Source: three-view drawing plus pictorial views. Frame: mm from the lowest corner of the part. A direction names the side the tool comes from. Coordinates: 2 decimals unless noted, no trailing zeros. Order: outer loops, then holes, each group sorted by start corner. A loop starts at its lowest first (then second) coordinate and runs counter-clockwise, first axis right, second up. Notation, with made-up numbers: (22.5, 21) - (44.5, 21) arc R21 cw to (44.5, 48) - close; hole circle Ø3 at (14, 87). An arc over 180 degrees is marked (long way). One line per question, with ' | ' between items.
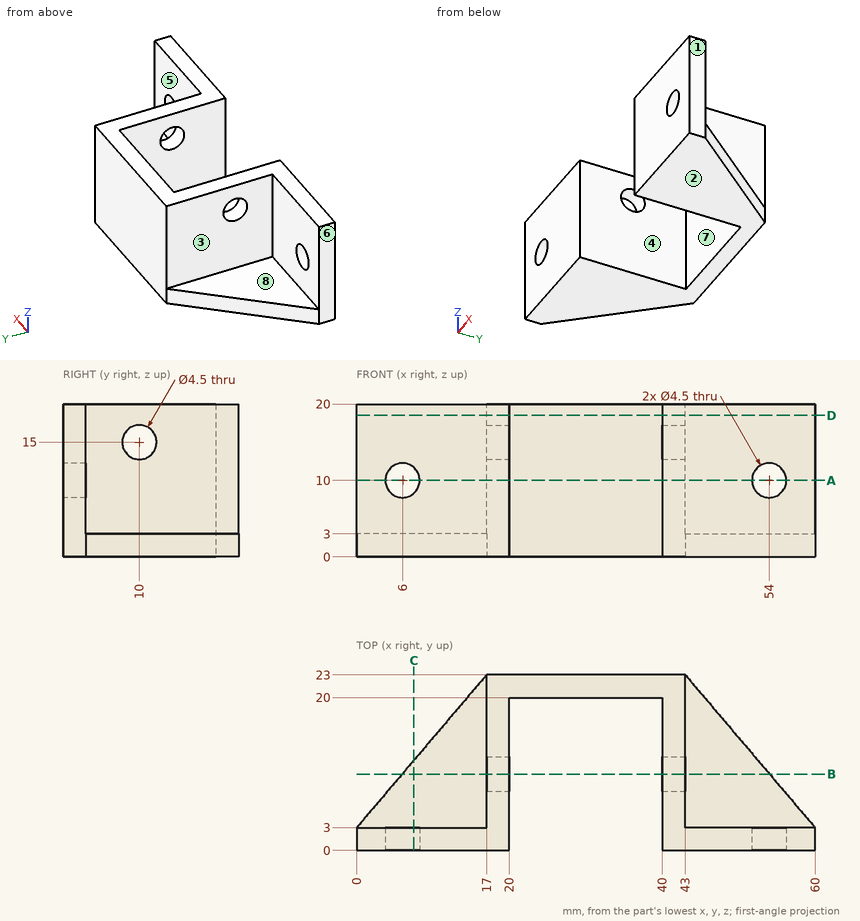
Item 1: Ray query, line 1 (X direction, y = 0.9, z = 10); line 2 (X direction, y = 8.75, z = 11.5); line 3 (Y direction, x = 40.75, z = 15). Return the intervals inside material, ascending.
Data:
line 1: 0 to 3.75, 8.25 to 20, 40 to 51.75, 56.25 to 60 | line 2: 17 to 20, 40 to 43 | line 3: 0 to 7.75, 12.25 to 23
Item 2: Access query for the marked faces 5, 6, 7 and 8. Directions: +Z, -Z, +X, -X, +Y, -Y. A direction counts if a zero-diameter tool reaches every point of the face in a straight line with its end or side. Return the directions, or none.
Data:
face 5: +Z, +X, +Y | face 6: +Z, -Z, -X, +Y, -Y | face 7: +Z, -Z, -Y | face 8: +Z, -X, +Y
Item 3: Section A-A on z = 10. Return the cut outline in (x, y).
Data:
outline: (0, 0) - (3.75, 0) - (3.75, 3) - (0, 3) - close; (8.25, 0) - (20, 0) - (20, 20) - (40, 20) - (40, 0) - (51.75, 0) - (51.75, 3) - (43, 3) - (43, 23) - (17, 23) - (17, 3) - (8.25, 3) - close; (56.25, 0) - (60, 0) - (60, 3) - (56.25, 3) - close
Item 4: Section D-D on z = 18.5. Return the cut outline in (x, y).
Data:
outline: (0, 0) - (20, 0) - (20, 20) - (40, 20) - (40, 0) - (60, 0) - (60, 3) - (43, 3) - (43, 23) - (17, 23) - (17, 3) - (0, 3) - close
Item 5: Contact query for flat-ended pins moving along their axis: P1, Ø12, axis at y = 12.5, z = 12, coming from the +X side; P2, Ø5, axis at x = 4.5, z = 8, coming from the +Y side; P3, Ø8.5, axis at x = 8.5, y = 14, coming from the +Z side; P4, Ø3.5, axis at y = 10, z = 15, coming from the +X side. Output: stop coordinate, or through.
Data:
P1: x = 43 | P2: y = 3 | P3: z = 3 | P4: through
Item 6: Section C-C on x = 7.5. Return the cut outline in (y, z).
Data:
outline: (0, 0) - (11.82, 0) - (11.82, 3) - (3, 3) - (3, 8.32) - (0, 8.32) - close; (0, 11.68) - (3, 11.68) - (3, 20) - (0, 20) - close
Item 7: Draft query along X for the marked faces 1, 2, 3 and 4. Return one class per face: released by +X, released by -X, zero draft, split by the parting line, or undercut.
Data:
face 1: released by +X | face 2: zero draft | face 3: released by -X | face 4: undercut
Item 8: Section B-B on y = 10. Return the cut outline in (x, z), and give its area (3 significant figures).
Data:
outline: (5.95, 0) - (20, 0) - (20, 12.75) - (17, 12.75) - (17, 3) - (5.95, 3) - close; (17, 17.25) - (20, 17.25) - (20, 20) - (17, 20) - close; (40, 0) - (54.05, 0) - (54.05, 3) - (43, 3) - (43, 12.75) - (40, 12.75) - close; (40, 17.25) - (43, 17.25) - (43, 20) - (40, 20) - close | area: 159 mm^2
